The model under review builds one solid part; all positions refer to its coordinate system, in mm. Face numbers are marked on the shaded views. A direction names the side the tool comes from. Round coordinates to 2 decimals unless told otherwise and drop trailing zeros. Order: outer loops, then holes, each group sorted by start corner. A loop starts at its lowest first (then second) coordinate and runs counter-clockwise, first axis right, second up.
```python
from build123d import *

# Parameters (mm, degrees)
F0_W      = 457.2
F0_H      = 406.4
F1_DEPTH  = 1219.2
F2_W      = 431.8
F2_H      = 402.8296259509
F3_DEPTH  = 152.4
F4_R      = 6.7564
F5_W      = 431.8
F5_H      = 304.8
F6_DEPTH  = 355.6
F7_W      = 431.8
F7_H      = 254
F7_H_2    = 203.2
F8_DEPTH  = 355.6
F9_R      = 6.1321024484
F10_W     = 219.456
F10_H     = 130.556
F11_DEPTH = 203.2
F12_R     = 5.08


with BuildPart() as f1:
    # F0 (on Top) → F1 (new body)
    with BuildSketch(Plane.XY):
        with Locations((-6.7284821169, -163.7329156511)):
            Rectangle(F0_W, F0_H)
    extrude(amount=-F1_DEPTH)

    # F2 (on face) → F3 (cut)
    with BuildSketch(Plane.XY):
        with Locations((-6.7284821169, -174.6477286265)):
            Rectangle(F2_W, F2_H)
    extrude(amount=-F3_DEPTH, mode=Mode.SUBTRACT)

    # F4
    f4_edges = [f1.edges().sort_by_distance(p)[0] for p in [
        (209.171518, -170.082916, -152.4),
        (-6.728482, 26.767084, -152.4),
        (209.171518, 26.767084, -76.2),
        (209.171518, -366.932916, -76.2),
        (209.171518, -170.082916, 0),
        (215.521518, -366.932916, 0),
        (-222.628482, -170.082916, -152.4),
        (-222.628482, 26.767084, -76.2),
        (-6.728482, -366.932916, -152.4),
        (-222.628482, -366.932916, -76.2),
        (-222.628482, -170.082916, 0),
        (-228.978482, -366.932916, 0),
        (-6.728482, 26.767084, 0),
    ]]
    fillet(f4_edges, radius=F4_R)

    # F5 (on face) → F6 (cut)
    with BuildSketch(Plane.XZ.offset(366.9329156511)):
        with Locations((-6.7284821169, -1054.1)):
            Rectangle(F5_W, F5_H)
    extrude(amount=-F6_DEPTH, mode=Mode.SUBTRACT)

    # F7 (on face) → F8 (cut)
    with BuildSketch(Plane.XZ.offset(366.9329156511)):
        with Locations((-6.7284821169, -762)):
            Rectangle(F7_W, F7_H)
        with Locations((-6.7284821169, -520.7)):
            Rectangle(F7_W, F7_H_2)
        Polygon((-121.0284821169, -298.8564), (-121.0284821169, -159.1564), (-222.6284821169, -159.1564), (-222.6284821169, -406.4), (209.1715178831, -406.4), (209.1715178831, -159.1564), (107.5715178831, -159.1564), (107.5715178831, -298.8564), align=None)
    extrude(amount=-F8_DEPTH, mode=Mode.SUBTRACT)

    # F9
    f9_edges = [f1.edges().sort_by_distance(p)[0] for p in [
        (-222.628482, -366.932916, -520.7),
        (209.171518, -366.932916, -520.7),
        (-222.628482, -366.932916, -282.7782),
        (209.171518, -366.932916, -282.7782),
        (209.171518, -366.932916, -762),
        (-222.628482, -366.932916, -762),
        (-222.628482, -366.932916, -1054.1),
        (209.171518, -366.932916, -1054.1),
        (-6.728482, -366.932916, -1206.5),
        (-6.728482, -366.932916, -889),
        (-6.728482, -366.932916, -901.7),
        (-6.728482, -366.932916, -635),
        (-6.728482, -366.932916, -622.3),
        (-6.728482, -366.932916, -419.1),
        (-6.728482, -366.932916, -406.4),
    ]]
    fillet(f9_edges, radius=F9_R)

    # F10 (on face) → F11 (cut)
    with BuildSketch(Plane.XZ.offset(366.9329156511)):
        with Locations((-6.7284821169, -229.0064)):
            Rectangle(F10_W, F10_H)
    extrude(amount=-F11_DEPTH, mode=Mode.SUBTRACT)

    # F12
    f12_edges = [f1.edges().sort_by_distance(p)[0] for p in [
        (-235.328482, -366.932916, -612.9782),
        (221.871518, -366.932916, -612.9782),
        (221.871518, -160.354716, 0),
        (-235.328482, -160.354716, 0),
        (221.871518, -364.954012, -1.978904),
        (-235.328482, -364.954012, -1.978904),
    ]]
    fillet(f12_edges, radius=F12_R)


solid = f1.part
```
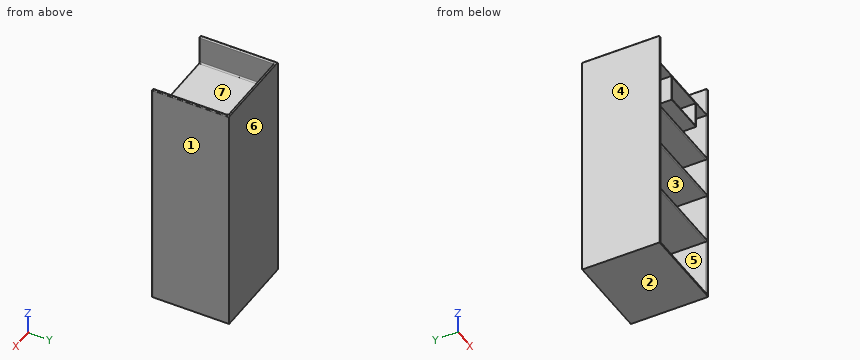
(1) Consider section A-A (y = -71). State how many separate pieces and enclosed holes the cut face has, and give its area (3 significant figures).
Data:
separate pieces: 1
enclosed holes: 4
area: 87,700 mm2
(2) To check wall thickness, follow probe 1 along Z at (x, y) = (-98, -295); probe 2 along Z at (x, y) = (146.5, -304.5); probe 3 along Z at (x, y) = (-22, -82.5). State the ranges of each line that lie inside material, in increasing order.
Data:
probe 1: z = -1219.2 to -1206.5, -901.7 to -889, -635 to -622.3, -419.1 to -406.4, -298.86 to -294.28, -163.73 to -152.4
probe 2: z = -1219.2 to -1206.5, -901.7 to -889, -635 to -622.3, -419.1 to -406.4, -159.16 to -152.4
probe 3: z = -1219.2 to -1206.5, -901.7 to -889, -635 to -622.3, -419.1 to -406.4, -298.86 to -152.4
(3) Draft analysis for pull direction X (two halves, no side actions). For the marked faces 1, 2, 3 and 4, state which applies: pulls with the +X half, pulls with the -X half, needs draft (parallel to the pull), parting line crosses it, or undercut.
Data:
face 1: pulls with the +X half
face 2: needs draft
face 3: undercut
face 4: pulls with the -X half
(4) For the marked faces 5, 6 and 7, list the 3-axis set-ups (+Z, -Z, +X, -X, +Y, -Y) from which the entire face can be reached by the end or side of a thin tool; tool diameter is ignored.
Data:
face 5: -Y
face 6: +Z, -Z, +X, -X, +Y
face 7: +Z, -Y
(5) Consider section B-B (z = -268). Write out the cut boundary in (x, y).
Data:
outline: (-235.33, -361.85) arc R5.08 ccw to (-230.25, -366.93) - (-228.76, -366.93) arc R6.13 ccw to (-222.63, -360.8) - (-222.63, -11.33) - (-121.03, -11.33) - (-121.03, -366.93) - (-116.46, -366.93) - (-116.46, -163.73) - (103, -163.73) - (103, -366.93) - (107.57, -366.93) - (107.57, -11.33) - (209.17, -11.33) - (209.17, -360.8) arc R6.13 ccw to (215.3, -366.93) - (216.79, -366.93) arc R5.08 ccw to (221.87, -361.85) - (221.87, 39.47) - (-235.33, 39.47) - close
(6) Insertion check: pin 1 (8 mm diameter, centred on x = -189, y = -8.5, fed in from +Z); pin 2 (5 mm diameter, centred on x = 156, z = -192, fed in from -Y). Each pin has a flat end and moves straight along its axis. Give the tip position at first contact, or say it passes through.
Data:
pin 1: stops at z = -152.4
pin 2: stops at y = -11.33
